Part model, mm, in its own coordinate system. Give positions to 0.01 mm unless a question says otherwise; leave off trailing zeros. Loops run counter-clockwise (first coordinate to the right, second up) from the corner with the lowest first, then second, coordinate; pieces in that order, holes last. Notation, with made-up numbers: M 82.5,-28 L 102.5,-28 A8 ccw 102.5,-14 Z; hole C 60.5,36 d1. An arc over 180 degrees is marked long. Answer in a Markdown table with one row per item.
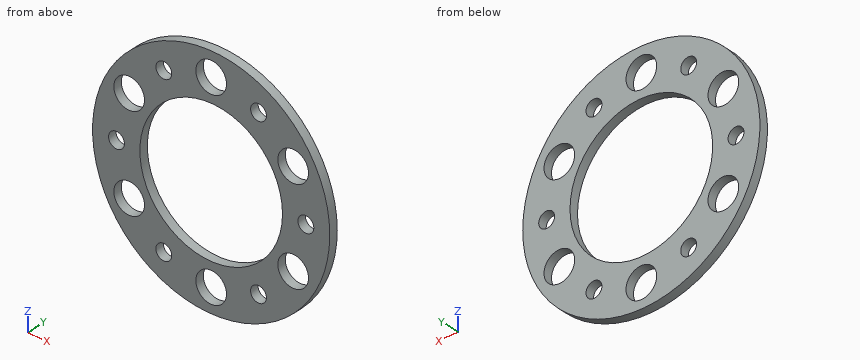
from build123d import *

# Parameters (mm, degrees)
SKETCH1_R             = 16.891
SKETCH1_R_2           = 10.16
BOSS_EXTRUDE1_DEPTH   = 1.27
SKETCH2_R             = 2.1844
CUT_EXTRUDE1_DEPTH    = 2.27
F_4_40_TAPPED_HOLE1_D = 2.2606


with BuildPart() as part:
    # Sketch1 → Boss-Extrude1 (new body)
    with BuildSketch(Plane(origin=(0, 0, 0), x_dir=(1, 0, 0), z_dir=(0, 1, 0))):
        Circle(SKETCH1_R)
        Circle(SKETCH1_R_2, mode=Mode.SUBTRACT)
    extrude(amount=BOSS_EXTRUDE1_DEPTH)

    # Sketch2 → Cut-Extrude1 (cut, through all)
    with BuildSketch(Plane(origin=(0, 1.27, 0), x_dir=(1, 0, 0), z_dir=(0, 1, 0))):
        with Locations((0, 13.4874)):
            Circle(SKETCH2_R)
        with Locations((-11.680431031, 6.7437)):
            Circle(SKETCH2_R)
        with Locations((-11.680431031, -6.7437)):
            Circle(SKETCH2_R)
        with Locations((0, -13.4874)):
            Circle(SKETCH2_R)
        with Locations((11.680431031, -6.7437)):
            Circle(SKETCH2_R)
        with Locations((11.680431031, 6.7437)):
            Circle(SKETCH2_R)
    extrude(amount=-CUT_EXTRUDE1_DEPTH, mode=Mode.SUBTRACT)

    # #4-40 Tapped Hole1 (through all)
    with Locations(Plane(origin=(0, 1.27, 0), x_dir=(1, 0, 0), z_dir=(0, 1, 0))):
        with Locations((0, 0), (-6.7437, 11.680431031), (6.7437, 11.680431031), (13.4874, 0), (6.7437, -11.680431031), (-6.7437, -11.680431031), (-13.4874, 0)):
            Hole(F_4_40_TAPPED_HOLE1_D / 2)


solid = part.part
(1) Saw through at B-B (z = -8.5). Write the cut outline in (x, y).
Recorded:
| item | result |
|---|---|
| outline | M -14.6,0 L -12.98,0 L -12.98,1.27 L -14.6,1.27 Z; M -10.38,0 L -5.57,0 L -5.57,1.27 L -10.38,1.27 Z; M 5.57,0 L 10.38,0 L 10.38,1.27 L 5.57,1.27 Z; M 12.98,0 L 14.6,0 L 14.6,1.27 L 12.98,1.27 Z |
(2) Drill centre lines: line 1 along X through (y, z) = (0.2, -0.5); line 2 along X through (y, z) = (0.65, 5.5); line 3 along Z through (x, y) = (7.5, 0.1). Where is each one in solid material? Low to high.
Recorded:
| item | result |
|---|---|
| line 1 | x = -16.88 to -14.5, -12.47 to -10.15, 10.15 to 12.47, 14.5 to 16.88 |
| line 2 | x = -15.97 to -13.48, -9.88 to -8.54, 8.54 to 9.88, 13.48 to 15.97 |
| line 3 | z = -15.13 to -12.52, -10.84 to -6.85, 6.85 to 10.84, 12.52 to 15.13 |
(3) Saw through at A-A (x = 0). Write the cut outline in (y, z), plus the area to 3 significant figures.
Recorded:
| item | result |
|---|---|
| outline | M 0,-16.89 L 1.27,-16.89 L 1.27,-15.67 L 0,-15.67 Z; M 0,-11.3 L 1.27,-11.3 L 1.27,-10.16 L 0,-10.16 Z; M 0,10.16 L 1.27,10.16 L 1.27,11.3 L 0,11.3 Z; M 0,15.67 L 1.27,15.67 L 1.27,16.89 L 0,16.89 Z |
| area | 6.00 mm^2 |
(4) Saw through at D-D (x = -11). Write the cut outline in (y, z), plus the area to 3 significant figures.
Recorded:
| item | result |
|---|---|
| outline | M 0,-12.82 L 1.27,-12.82 L 1.27,-8.82 L 0,-8.82 Z; M 0,-4.67 L 1.27,-4.67 L 1.27,4.67 L 0,4.67 Z; M 0,8.82 L 1.27,8.82 L 1.27,12.82 L 0,12.82 Z |
| area | 22.0 mm^2 |
(5) Saw through at C-C (z = -15). Write the cut outline in (x, y), plus the area to 3 significant figures.
Recorded:
| item | result |
|---|---|
| outline | M -7.77,0 L -1.58,0 L -1.58,1.27 L -7.77,1.27 Z; M 1.58,0 L 7.77,0 L 7.77,1.27 L 1.58,1.27 Z |
| area | 15.7 mm^2 |
